```python
from build123d import *

# Parameters (mm, degrees)
F0_R     = 12.7
F1_DEPTH = 21.59
F2_SIZE  = 2.54
F4_D     = 4.0386
F4_DEPTH = 11.90625
F4_TIP   = 1.213317848


with BuildPart() as f1:
    # F0 (on Front) → F1 (new body)
    with BuildSketch(Plane.XZ):
        Circle(F0_R)
    extrude(amount=F1_DEPTH)

    # F2
    f2_edges = [f1.edges().sort_by_distance(p)[0] for p in [
        (-12.7, -21.59, 0),
    ]]
    chamfer(f2_edges, length=F2_SIZE)

    # F4
    with Locations(Plane(origin=(0, 0, 0), x_dir=(-1, 0, 0), z_dir=(0, 1, 0))):
        with Locations((0, 0)):
            Hole(F4_D / 2, depth=F4_DEPTH)
            with Locations((0, 0, -(F4_DEPTH + F4_TIP / 2))):  # 118° drill point
                Cone(0, F4_D / 2, F4_TIP, mode=Mode.SUBTRACT)


solid = f1.part
```
Source: CAD feature listing. Evaluate the final solid. Frame: model axes, mm. Give positions to 0.01 mm unless a question says otherwise; leave off trailing zeros. Loops run counter-clockwise (first coordinate to the right, second up) from the corner with the lowest first, then second, coordinate; pieces in that order, holes last. Notation, with made-up numbers: M 62,89.25 L 89,89.25 A18 cw 89,115.25 Z; hole C 23.25,-31 d1. An arc over 180 degrees is marked long. Put each result on its own line as item: value.
Q1. Section A-A (y = -9.5). Return the cut outline in (x, z), and give its area (3 significant figures).
Response values:
outline: C 0,0 d25.4; hole C 0,0 d4.04
area: 494 mm²
Q2. Line query: probe 1 along Z at (x, y) = (0, -3.75); probe 2 along X at (y, z) = (-20.25, -0.25); probe 3 along X at (y, z) = (-10.5, -1.25). Output: solid intervals per line, ascending. Write a range as [from, to].
Response values:
probe 1: z = [-12.7, -2.02], [2.02, 12.7]
probe 2: x = [-11.5, 11.5]
probe 3: x = [-12.64, -1.59], [1.59, 12.64]
Q3. Mould query, pull axis Z, two halves, no side actions, for faces 1 (the cylindrical face through (1.926, -6.036, 0.607)), 2 (the flat face through (3, 0, 0)), 3 (the cylindrical face through (-2.75, -9.39, -12.4)). Classes: released by +Z, released by -Z, zero draft, split by the parting line, or undercut.
Response values:
face 1: undercut
face 2: zero draft
face 3: split by the parting line
Q4. Pin query (flat end, axial travel): P1, Ø1, axis at x = 3.5, y = -12, coming from the +Z side; P2, Ø1.5, axis at y = -11.5, z = -7.5, coming from the +X side; P3, Ø8, axis at x = -6.5, y = -11, coming from the -Z side. Return the tip coordinate at first contact, or that it passes through.
Response values:
P1: stops at z = 12.34
P2: stops at x = 10.76
P3: stops at z = -12.45
